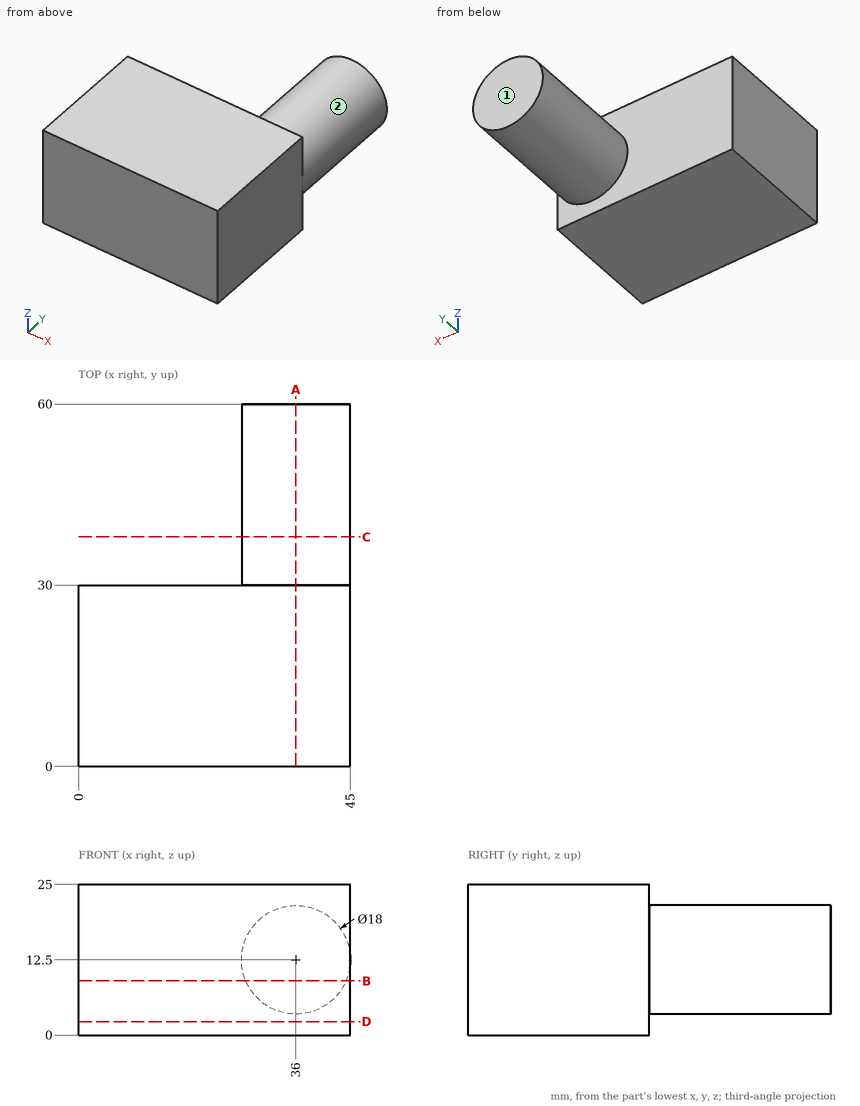
The drawing under review shows one solid part. Ordinate dimensions are in mm from its lowest x, y, z. A direction names the side the tool comes from. Round coordinates to 2 decimals unless told otherwise and drop trailing zeros. Write each loop counter-clockwise with the first axis right and the second up, starting at its lowest first coordinate (ties: lowest second). Pieces come first, ordered by that corner, then holes. Notation, with made-up numbers: M 22.25,87 L 28.25,87 A15 cw 28.25,94 Z; hole C 16.5,89.25 d7. An arc over 180 degrees is marked long. One line per item, written item: value. Start each with the question number.
(1) Wall thickness on line 1 (Y direction, x = 23.5, z = 18.5); line 2 (Z direction, x = 36, y = 47); line 3 (Z direction, x = 32.5, y = 47.5): over which ranges is each line inside the solid? List them lowest first.
(2) Insertion check: pin 1 (5 mm diameter, centred on x = 6, z = 17, fed in from +Y). The pin has a flat end and moves straight along its axis. Give the tip position at first contact, or say it passes through.
(3) We need section C-C (y = 38). Give the boundary of the cut face in (x, z).
(4) We need section D-D (z = 2.25). Give the boundary of the cut face in (x, y), and give its area (3 significant figures).
(5) Machinability: for the marked faces 1 and 2, which of the approach directions +Z, -Z, +X, -X, +Y, -Y give a long, thin tool a straight path to every point of the face, cutting with its end or side? Answer none if there is none.
(6) We need section A-A (x = 36). Give the boundary of the cut face in (y, z), and give its area (3 significant figures).
(7) We need section B-B (z = 9). Give the boundary of the cut face in (x, y).
Result:
1. line 1: 0 to 30
1. line 2: 3.5 to 21.5
1. line 3: 4.21 to 20.79
2. pin 1: y = 30
3. outline: C 36,12.5 d18
4. outline: M 0,0 L 45,0 L 45,30 L 0,30 Z
4. area: 1,350 mm²
5. face 1: +Z, -Z, +X, -X, +Y
5. face 2: +Y
6. outline: M 0,0 L 30,0 L 30,3.5 L 60,3.5 L 60,21.5 L 30,21.5 L 30,25 L 0,25 Z
6. area: 1,290 mm²
7. outline: M 0,0 L 45,0 L 45,30 L 44.29,30 L 44.29,60 L 27.71,60 L 27.71,30 L 0,30 Z
